from build123d import *

# Parameters (mm, degrees)
F0_W     = 53
F0_H     = 53
F1_DEPTH = 3
F3_DEPTH = 1.3
F4_W     = 33
F4_H     = 3
F5_DEPTH = 3
F6_R     = 1.8
F7_R     = 1.5


with BuildPart() as f1:
    # F0 (on Top) → F1 (new body)
    with BuildSketch(Plane.XY):
        with Locations((0.098538, 0.495021)):
            Rectangle(F0_W, F0_H)
    extrude(amount=F1_DEPTH)

    # F2 (on face) → F3 (cut)
    with BuildSketch(Plane.XY.offset(3)):
        with BuildLine():
            Line((-24.401462, -23.004979), (-24.401462, -21.454979))
            ThreePointArc((-24.401462, -21.454979), (-25.497478, -24.100995), (-22.851462, -23.004979))
            Line((-22.851462, -23.004979), (-24.401462, -23.004979))
        make_face()
        with BuildLine():
            ThreePointArc((26.148538, -23.004979), (25.694553, -21.908964), (24.598538, -21.454979))
            Line((24.598538, -21.454979), (24.598538, -23.004979))
            Line((24.598538, -23.004979), (23.048538, -23.004979))
            ThreePointArc((23.048538, -23.004979), (24.598538, -24.554979), (26.148538, -23.004979))
        make_face()
        with BuildLine():
            Line((24.598538, -23.004979), (24.598538, -21.454979))
            ThreePointArc((24.598538, -21.454979), (23.502522, -21.908964), (23.048538, -23.004979))
            Line((23.048538, -23.004979), (24.598538, -23.004979))
        make_face()
        with BuildLine():
            ThreePointArc((-22.851462, -23.004979), (-23.305447, -21.908964), (-24.401462, -21.454979))
            Line((-24.401462, -21.454979), (-24.401462, -23.004979))
            Line((-24.401462, -23.004979), (-22.851462, -23.004979))
        make_face()
    extrude(amount=-F3_DEPTH, mode=Mode.SUBTRACT)

    # F4 (on face) → F5 (join)
    with BuildSketch(Plane.XY.offset(3)):
        with Locations((0.098538, 25.495021)):
            Rectangle(F4_W, F4_H)
    extrude(amount=F5_DEPTH)

    # F6
    f6_edges = [f1.edges().sort_by_distance(p)[0] for p in [
        (0.098538, 26.995021, 6),
    ]]
    fillet(f6_edges, radius=F6_R)

    # F7
    f7_edges = [f1.edges().sort_by_distance(p)[0] for p in [
        (26.598538, -26.004979, 1.5),
        (-26.401462, -26.004979, 1.5),
    ]]
    fillet(f7_edges, radius=F7_R)


solid = f1.part
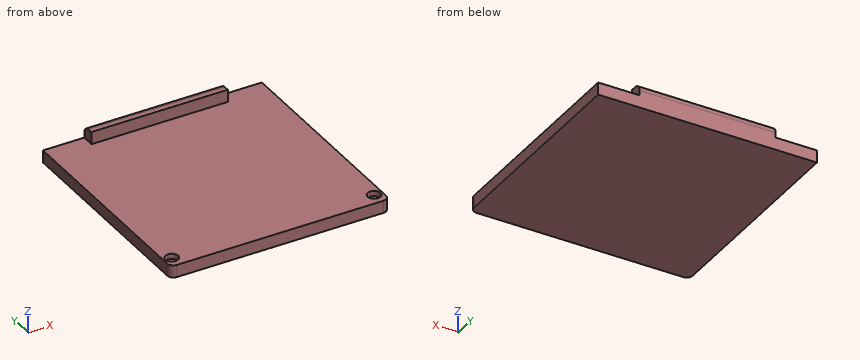
Geometry: final body of the model. Coordinates: model frame, mm. Coordinates: 2 decimals unless noted, no trailing zeros. Loops run counter-clockwise (first coordinate to the right, second up) from the corner with the lowest first, then second, coordinate; pieces in that order, holes last. Notation, with made-up numbers: (28.5, 86) - (40.5, 86) arc R28 ccw to (40.5, 119) - close; hole circle Ø3 at (-39, -30). An arc over 180 degrees is marked (long way). Put each result on its own line as item: value. Start each with the question number.
Q1. Cut plane C-C, the plane x = 18. Return loops of the section in (y, z), and give its area (3 significant figures).
Q2. Line query: line 1 (Y direction, x = 24.5, z = 1.75); line 2 (Z direction, x = 16, y = -18); line 3 (Y direction, x = 12, z = 3.25). Output: solid intervals per line, ascending.
Q3. Pin query (flat end, axial travel): pin 1 Ø0.9 at (y, z) = (26, 4) entering from +X; pin 2 Ø0.9 at (y, z) = (25, 5) entering from -X; pin 3 Ø2.5 at (x, y) = (24.5, -23) entering from +Z. Return the tip coordinate at first contact, or that it passes through.
Q4. Cut plane B-B, the plane y = -11.5. Return loops of the section in (x, z), and give its area (3 significant figures).
Q5. Cut plane A-A, the plane x = 10.5. Return loops of the section in (y, z), and give its area (3 significant figures).
Filled sheet:
1. outline: (-26, 0) - (27, 0) - (27, 3) - (-26, 3) - close
1. area: 159 mm²
2. line 1: -26 to -24.55, -21.46 to 27
2. line 2: 0 to 3
2. line 3: 24 to 27
3. pin 1: x = 16.6
3. pin 2: x = -16.4
3. pin 3: z = 1.7
4. outline: (-26.4, 0) - (26.6, 0) - (26.6, 3) - (-26.4, 3) - close
4. area: 159 mm²
5. outline: (-26, 0) - (27, 0) - (27, 4.2) arc R1.8 ccw to (25.2, 6) - (24, 6) - (24, 3) - (-26, 3) - close
5. area: 167 mm²
